Read the model definition and answer for the solid it produces. Units are mm, in the model's axes. Face numbers are marked on the shaded views. A direction names the side the tool comes from. Give positions to 0.01 mm unless a question says otherwise; leave off trailing zeros. Loops run counter-clockwise (first coordinate to the right, second up) from the corner with the lowest first, then second, coordinate; pieces in that order, holes last. Notation, with made-up numbers: (43.5, -28.75) - (84.5, -28.75) arc R23 cw to (84.5, -5.75) - close; hole circle Ø9 at (81, -4.75). An arc over 180 degrees is marked (long way). Write item = value, one per line.
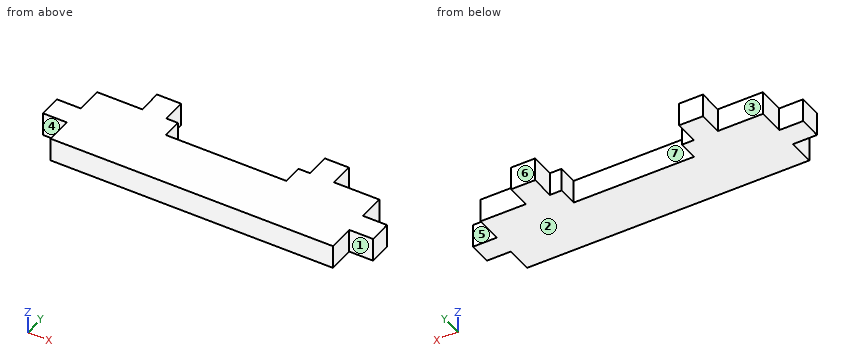
```python
from build123d import *

# Parameters (mm, degrees)
BOSS_EXTRUDE1_DEPTH = 3.125


with BuildPart() as part:
    # Sketch2 → Boss-Extrude1 (new body)
    with BuildSketch(Plane.XY):
        Polygon((0, -6.59), (18.735, -6.59), (18.735, -3.09), (21.915, -3.09), (21.915, -0.09), (18.735, -0.09), (18.735, 3.41), (12.735, 3.41), (12.735, 6.59), (9.555, 6.59), (9.555, 3.41), (7.995, 3.41), (7.995, 0.81), (0.569270121, 0.81), (0, 0.81), align=None)
    boss_extrude1 = extrude(amount=BOSS_EXTRUDE1_DEPTH)

    # Mirror1: Boss-Extrude1 across plane
    add(boss_extrude1.mirror(Plane(origin=(0, -6.59, 3.125), x_dir=(0, 0, 1), z_dir=(1, 0, 0))))


solid = part.part
```
1) A cutting plane is placed at B-B on z = 2.3. Determine the outline of the cut face in (x, y) (3 decimals).
Output:
outline = (-21.915, -3.09) - (-18.735, -3.09) - (-18.735, -6.59) - (18.735, -6.59) - (18.735, -3.09) - (21.915, -3.09) - (21.915, -0.09) - (18.735, -0.09) - (18.735, 3.41) - (12.735, 3.41) - (12.735, 6.59) - (9.555, 6.59) - (9.555, 3.41) - (7.995, 3.41) - (7.995, 0.81) - (-7.995, 0.81) - (-7.995, 3.41) - (-9.555, 3.41) - (-9.555, 6.59) - (-12.735, 6.59) - (-12.735, 3.41) - (-18.735, 3.41) - (-18.735, -0.09) - (-21.915, -0.09) - close
2) Each of these flat-tipped pins is pushed along its axis until it touches: P1, Ø1.6, axis at y = 1, z = 2.5, coming from the -X side (3 decimals); P2, Ø0.9, axis at x = -16, z = 1, coming from the +Y side; P3, Ø1.6, axis at x = -20, z = 2.5, coming from the -Y side. Where does it stop, or does it pass through?
Output:
P1 = -18.735
P2 = 3.41
P3 = -3.09
3) A cutting plane is placed at A-A on y = 2.75. Determine the outline of the cut face in (x, z) (3 decimals), then the cut area to 3 significant figures.
Output:
outline = (-18.735, 0) - (-7.995, 0) - (-7.995, 3.125) - (-18.735, 3.125) - close; (7.995, 0) - (18.735, 0) - (18.735, 3.125) - (7.995, 3.125) - close
area = 67.1 mm²
4) Find the intervals of material crossed by probe 1 along X at (y, z) = (2, 1.55) (3 decimals); probe 2 along X at (y, z) = (3.5, 1.75) (3 decimals); probe 3 along Y at (x, z) = (-18.5, 2.25), in increasing order.
Output:
probe_1 = -18.735 to -7.995, 7.995 to 18.735
probe_2 = -12.735 to -9.555, 9.555 to 12.735
probe_3 = -6.59 to 3.41
5) The mould has two halves that part along X. Classify the marked faces 6 and 7: pulls with the +X half, pulls with the -X half, needs draft (parallel to the pull), parting line crosses it, or undercut.
Output:
face_6 = needs draft
face_7 = undercut
6) A cutting plane is placed at D-D on x = -18. Determine the outline of the cut face in (y, z) (3 decimals), then the cut area to 4 significant figures.
Output:
outline = (-6.59, 0) - (3.41, 0) - (3.41, 3.125) - (-6.59, 3.125) - close
area = 31.25 mm²
7) A cutting plane is placed at C-C on y = 5.25. Determine the outline of the cut face in (x, z) (3 decimals).
Output:
outline = (-12.735, 0) - (-9.555, 0) - (-9.555, 3.125) - (-12.735, 3.125) - close; (9.555, 0) - (12.735, 0) - (12.735, 3.125) - (9.555, 3.125) - close
8) A tool of negligible diameter and unlimited length cuts with its end or side. For the marked faces 1, 2, 3, 4 and 5, from which of +Z, -Z, +X, -X, +Y, -Y can it reach the whole face along a straight path? Write none if from no direction.
Output:
face_1 = +Z, -Z, +X, -Y
face_2 = -Z, +X, -X, +Y, -Y
face_3 = +Z, -Z, -X, +Y
face_4 = +Z, -Z, -X, -Y
face_5 = +Z, -Z, +X, +Y
